Here's how the part is built. I have some questions about the finished solid (model axes, mm). Face numbers are marked on the shaded views. A direction names the side the tool comes from. Coordinates: 2 decimals unless noted, no trailing zeros. Write each loop counter-clockwise with the first axis right and the second up, starting at its lowest first coordinate (ties: lowest second). Pieces come first, ordered by that corner, then holes.
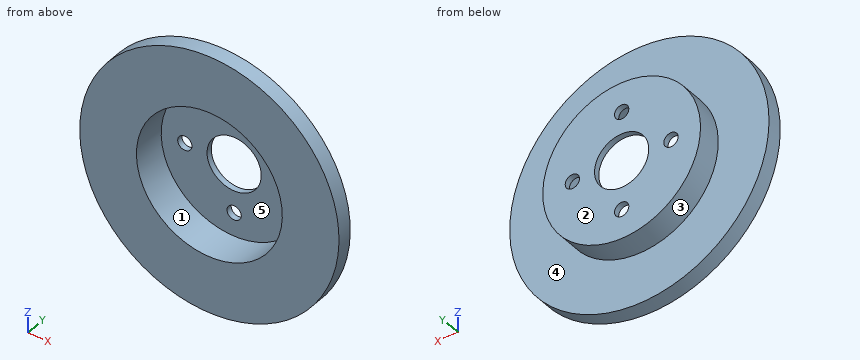
```python
from build123d import *

# Parameters (mm, degrees)
F3_D = 14.5


with BuildPart() as f1:
    # F0 (on Right) → F1 (revolve)
    with BuildSketch(Plane.YZ):
        Polygon((0, 74), (0, 27.5), (6, 27.5), (6, 80), (-19.2, 80), (-19.2, 131.5), (-35.2, 131.5), (-35.2, 74), align=None)
    revolve(axis=Axis((0, -66.1122447776, 0), (0, -1, 0)))

    # F3 (through all)
    with Locations(Plane(origin=(0, 6, 0), x_dir=(-1, 0, 0), z_dir=(0, 1, 0))):
        with Locations((0, 50), (50, 0), (0, -50), (-50, 0)):
            Hole(F3_D / 2)


solid = f1.part
```
1) Imagine slicing it at B-B on x = 0. Please give me the cut outline in (y, z), then the cut area to 3 significant figures.
Values follow:
outline: (-35.2, -131.5) - (-19.2, -131.5) - (-19.2, -80) - (6, -80) - (6, -57.25) - (0, -57.25) - (0, -74) - (-35.2, -74) - close; (-35.2, 74) - (0, 74) - (0, 57.25) - (6, 57.25) - (6, 80) - (-19.2, 80) - (-19.2, 131.5) - (-35.2, 131.5) - close; (0, -42.75) - (6, -42.75) - (6, -27.5) - (0, -27.5) - close; (0, 27.5) - (6, 27.5) - (6, 42.75) - (0, 42.75) - close
area: 2,530 mm2
2) We'd pull the mould along Z, two halves only. Please class the marked faces 3, 4 and 5: pulls with the +Z half, pulls with the -Z half, needs draft (parallel to the pull), parting line crosses it, or undercut.
Values follow:
face 3: parting line crosses it
face 4: needs draft
face 5: undercut
3) I need wall thicknesses on probe 1 along Z at (x, y) = (0, 2.6); probe 2 along Z at (x, y) = (0.5, -18.5); probe 3 along Z at (x, y) = (0, -21). Which ranges of each line are inside material? Lowest first, please.
Values follow:
probe 1: z = -80 to -57.25, -42.75 to -27.5, 27.5 to 42.75, 57.25 to 80
probe 2: z = -80 to -74, 74 to 80
probe 3: z = -131.5 to -74, 74 to 131.5
4) Imagine slicing it at A-A on z = 0. Please give me the cut outline in (x, y).
Values follow:
outline: (-131.5, -35.2) - (-74, -35.2) - (-74, 0) - (-57.25, 0) - (-57.25, 6) - (-80, 6) - (-80, -19.2) - (-131.5, -19.2) - close; (-42.75, 0) - (-27.5, 0) - (-27.5, 6) - (-42.75, 6) - close; (27.5, 0) - (42.75, 0) - (42.75, 6) - (27.5, 6) - close; (57.25, 0) - (74, 0) - (74, -35.2) - (131.5, -35.2) - (131.5, -19.2) - (80, -19.2) - (80, 6) - (57.25, 6) - close
5) On a 3-axis mill with a long thin cutter (end or side, diameter ignored), from which of +Z, -Z, +X, -X, +Y, -Y can I reach the whole of each face in a straight line? I mean the marked faces 1 and 2. Say none if no direction works.
Values follow:
face 1: -Y
face 2: +Z, -Z, +X, -X, +Y
6) Imagine slicing it at C-C on x = 48. Please give me the cut outline in (y, z).
Values follow:
outline: (-35.2, -122.43) - (-19.2, -122.43) - (-19.2, -64) - (6, -64) - (6, -6.97) - (0, -6.97) - (0, -56.32) - (-35.2, -56.32) - close; (-35.2, 56.32) - (0, 56.32) - (0, 6.97) - (6, 6.97) - (6, 64) - (-19.2, 64) - (-19.2, 122.43) - (-35.2, 122.43) - close
7) Will these pins go through, and if not, where does the flat tip stop? pin 1 (19 mm diameter, centred on x = 0, z = -50, fed in from -Y); pin 2 (11.5 mm diameter, centred on x = 0, z = 50, fed in from +Y); pin 3 (2 mm diameter, centred on x = -68.5, y = -14.5, fed in from -Z); pin 4 (1 mm diameter, centred on y = -5, z = -32.5, fed in from +X).
Values follow:
pin 1: stops at y = 0
pin 2: passes through
pin 3: stops at z = -42.94
pin 4: stops at x = 73.32
8) Imagine slicing it at D-D on y = -30. Please give me the cut outline in (x, z).
Values follow:
outline: circle Ø263 at (0, 0); hole circle Ø148 at (0, 0)
